```python
from build123d import *

# Parameters (mm, degrees)
SKETCH1_W           = 119.5324
SKETCH1_H           = 78.0034
BOSS_EXTRUDE1_DEPTH = 1.5875
CUT_EXTRUDE1_REACH  = 3.587
SKETCH2_R           = 2
SKETCH3_R           = 0.508
CUT_EXTRUDE2_DEPTH  = 1.5875
CUT_EXTRUDE4_REACH  = 3.587
LPATTERN1_COUNT     = 26
LPATTERN1_PITCH     = 2.54


with BuildPart() as part:
    # Sketch1 → Boss-Extrude1 (new body)
    with BuildSketch(Plane(origin=(0, 0, 0), x_dir=(1, 0, 0), z_dir=(0, 1, 0))):
        Rectangle(SKETCH1_W, SKETCH1_H)
    extrude(amount=BOSS_EXTRUDE1_DEPTH)

    # Sketch2 → Cut-Extrude1 (cut, up to next)
    with BuildSketch(Plane(origin=(0, 1.5875, 0), x_dir=(1, 0, 0), z_dir=(0, 1, 0)), mode=Mode.PRIVATE) as cut_extrude1_sk1:
        with Locations((-55.7657, 35.0012)):
            Circle(SKETCH2_R)
    cut_extrude1_tool1 = extrude(cut_extrude1_sk1.sketch, amount=-CUT_EXTRUDE1_REACH, mode=Mode.PRIVATE) & part.part
    add(cut_extrude1_tool1.solids().sort_by_distance((-55.7657, 1.5875, -35.0012))[0], mode=Mode.SUBTRACT)
    # Sketch2 → Cut-Extrude1 (cut, up to next)
    with BuildSketch(Plane(origin=(0, 1.5875, 0), x_dir=(1, 0, 0), z_dir=(0, 1, 0)), mode=Mode.PRIVATE) as cut_extrude1_sk2:
        with Locations((-55.7657, -35.0012)):
            Circle(SKETCH2_R)
    cut_extrude1_tool2 = extrude(cut_extrude1_sk2.sketch, amount=-CUT_EXTRUDE1_REACH, mode=Mode.PRIVATE) & part.part
    add(cut_extrude1_tool2.solids().sort_by_distance((-55.7657, 1.5875, 35.0012))[0], mode=Mode.SUBTRACT)
    # Sketch2 → Cut-Extrude1 (cut, up to next)
    with BuildSketch(Plane(origin=(0, 1.5875, 0), x_dir=(1, 0, 0), z_dir=(0, 1, 0)), mode=Mode.PRIVATE) as cut_extrude1_sk3:
        with Locations((55.7657, 35.0012)):
            Circle(SKETCH2_R)
    cut_extrude1_tool3 = extrude(cut_extrude1_sk3.sketch, amount=-CUT_EXTRUDE1_REACH, mode=Mode.PRIVATE) & part.part
    add(cut_extrude1_tool3.solids().sort_by_distance((55.7657, 1.5875, -35.0012))[0], mode=Mode.SUBTRACT)
    # Sketch2 → Cut-Extrude1 (cut, up to next)
    with BuildSketch(Plane(origin=(0, 1.5875, 0), x_dir=(1, 0, 0), z_dir=(0, 1, 0)), mode=Mode.PRIVATE) as cut_extrude1_sk4:
        with Locations((55.7657, -35.0012)):
            Circle(SKETCH2_R)
    cut_extrude1_tool4 = extrude(cut_extrude1_sk4.sketch, amount=-CUT_EXTRUDE1_REACH, mode=Mode.PRIVATE) & part.part
    add(cut_extrude1_tool4.solids().sort_by_distance((55.7657, 1.5875, 35.0012))[0], mode=Mode.SUBTRACT)

    # Sketch3 → Cut-Extrude2 (cut)
    with BuildSketch(Plane(origin=(0, 1.5875, 0), x_dir=(1, 0, 0), z_dir=(0, 1, 0))):
        with Locations((-31.7373, 36.758)):
            Circle(SKETCH3_R)
        with Locations((-31.7373, -36.758)):
            Circle(SKETCH3_R)
    cut_extrude2 = extrude(amount=-CUT_EXTRUDE2_DEPTH, mode=Mode.SUBTRACT)

    # Sketch11 → Cut-Extrude4 (cut, up to next)
    with BuildSketch(Plane(origin=(0, 1.5875, 0), x_dir=(1, 0, 0), z_dir=(0, 1, 0)), mode=Mode.PRIVATE) as cut_extrude4_sk1:
        with BuildLine():
            Line((-59.7662, 35.0012), (-59.7662, 39.0017))
            Line((-59.7662, 39.0017), (-55.7657, 39.0017))
            ThreePointArc((-55.7657, 39.0017), (-58.594480678, 37.829980678), (-59.7662, 35.0012))
        make_face()
    cut_extrude4_tool1 = extrude(cut_extrude4_sk1.sketch, amount=-CUT_EXTRUDE4_REACH, mode=Mode.PRIVATE) & part.part
    add(cut_extrude4_tool1.solids().sort_by_distance((-58.872617, 1.5875, -38.108117))[0], mode=Mode.SUBTRACT)
    # Sketch11 → Cut-Extrude4 (cut, up to next)
    with BuildSketch(Plane(origin=(0, 1.5875, 0), x_dir=(1, 0, 0), z_dir=(0, 1, 0)), mode=Mode.PRIVATE) as cut_extrude4_sk2:
        with BuildLine():
            Line((-59.7662, -39.0017), (-55.7657, -39.0017))
            ThreePointArc((-55.7657, -39.0017), (-58.594480678, -37.829980678), (-59.7662, -35.0012))
            Line((-59.7662, -35.0012), (-59.7662, -39.0017))
        make_face()
    cut_extrude4_tool2 = extrude(cut_extrude4_sk2.sketch, amount=-CUT_EXTRUDE4_REACH, mode=Mode.PRIVATE) & part.part
    add(cut_extrude4_tool2.solids().sort_by_distance((-58.872617, 1.5875, 38.108117))[0], mode=Mode.SUBTRACT)
    # Sketch11 → Cut-Extrude4 (cut, up to next)
    with BuildSketch(Plane(origin=(0, 1.5875, 0), x_dir=(1, 0, 0), z_dir=(0, 1, 0)), mode=Mode.PRIVATE) as cut_extrude4_sk3:
        with BuildLine():
            Line((59.7662, -35.0012), (59.7662, -39.0017))
            Line((59.7662, -39.0017), (55.7657, -39.0017))
            ThreePointArc((55.7657, -39.0017), (58.594480678, -37.829980678), (59.7662, -35.0012))
        make_face()
    cut_extrude4_tool3 = extrude(cut_extrude4_sk3.sketch, amount=-CUT_EXTRUDE4_REACH, mode=Mode.PRIVATE) & part.part
    add(cut_extrude4_tool3.solids().sort_by_distance((58.872617, 1.5875, 38.108117))[0], mode=Mode.SUBTRACT)
    # Sketch11 → Cut-Extrude4 (cut, up to next)
    with BuildSketch(Plane(origin=(0, 1.5875, 0), x_dir=(1, 0, 0), z_dir=(0, 1, 0)), mode=Mode.PRIVATE) as cut_extrude4_sk4:
        with BuildLine():
            Line((59.7662, 39.0017), (55.7657, 39.0017))
            ThreePointArc((55.7657, 39.0017), (58.594480678, 37.829980678), (59.7662, 35.0012))
            Line((59.7662, 35.0012), (59.7662, 39.0017))
        make_face()
    cut_extrude4_tool4 = extrude(cut_extrude4_sk4.sketch, amount=-CUT_EXTRUDE4_REACH, mode=Mode.PRIVATE) & part.part
    add(cut_extrude4_tool4.solids().sort_by_distance((58.872617, 1.5875, -38.108117))[0], mode=Mode.SUBTRACT)

    # LPattern1: Cut-Extrude2 ×26
    with Locations(*[(i * LPATTERN1_PITCH, 0, 0) for i in range(1, LPATTERN1_COUNT)]):
        add(cut_extrude2, mode=Mode.SUBTRACT)


solid = part.part
```
Could you check a few things on this model? Use its own coordinates, in mm. Round coordinates to 2 decimals unless told otherwise and drop trailing zeros. One line per question, with ' | ' between items. Start each with the question number.
(1) Thinking about a two-plate mould opening in Z: for faces 1 (the face through (-53.86, 0.8, 34.4)), 2 (the face through (-1, 1.588, -1)), 3 (the face through (58.563, 0.805, -37.861)), which applies, +Z half, -Z half, draft (parallel to the pull), parting line (faces both ways), or undercut?
(2) For P1, Ø0.6, axis at x = 3.82, z = 36.76, coming from the -Y side, with a flat end and sliding along its axis, tell me the tip position at first contact or that it passes through.
(3) Please list where these lines run through material, in increasing order: line 1 along X through (y, z) = (0.8, 35); line 2 along X through (y, z) = (1, 33.5); line 3 along Z through (x, y) = (-4, 1.35).
Geometry results:
1) face 1: undercut | face 2: draft | face 3: -Z half
2) P1: through
3) line 1: -59.77 to -57.77, -53.77 to 53.77, 57.77 to 59.77 | line 2: -59.77 to -57.09, -54.44 to 54.44, 57.09 to 59.77 | line 3: -39 to -37.22, -36.29 to 36.29, 37.22 to 39
